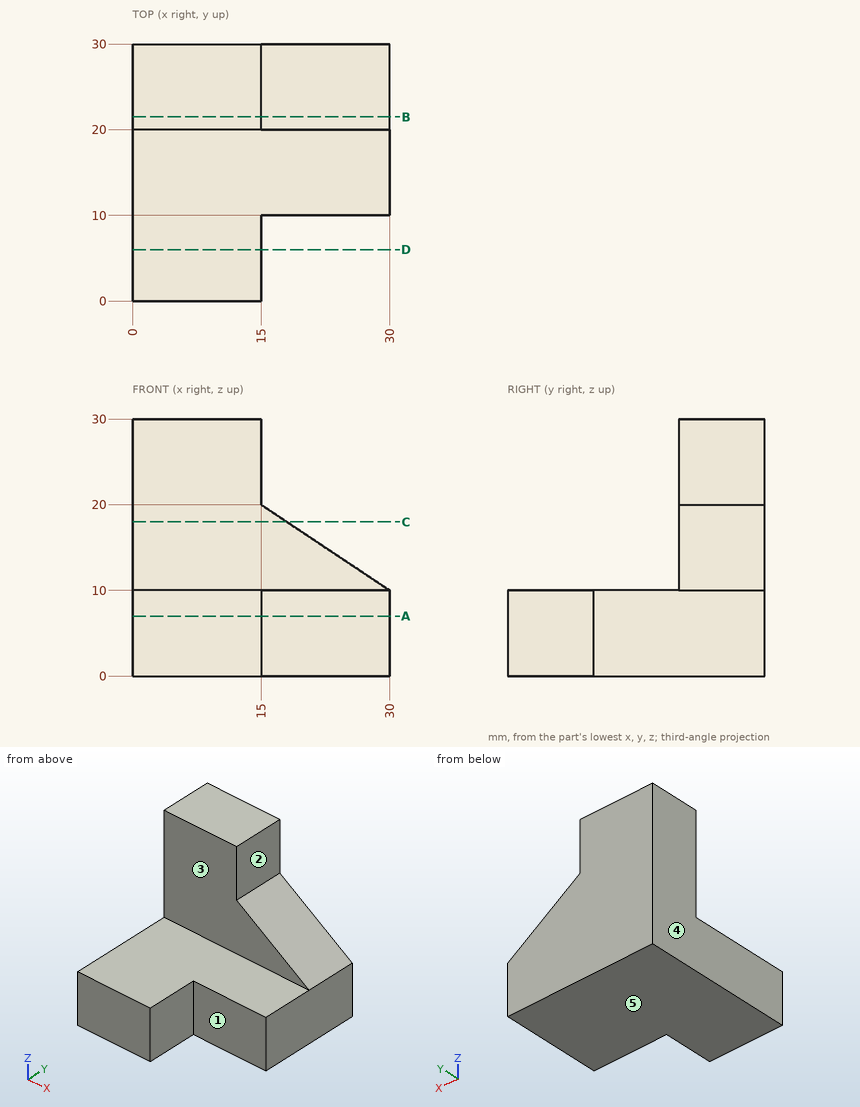
Design review of the part shown in the three views and the two pictorial views. Dimensions are in mm from the part's minimum x, y and z. A direction names the side the tool comes from. Give positions to 0.01 mm unless a question says otherwise; leave off trailing zeros. Loops run counter-clockwise (first coordinate to the right, second up) from the corner with the lowest first, then second, coordinate; pieces in that order, holes last. Notation, with made-up numbers: (4.5, 63.25) -> (21.5, 63.25) arc R9 ccw to (21.5, 79.25) -> close; hole circle Ø7 at (34.5, 63.5). An arc over 180 degrees is marked (long way). Put each result on its own line as item: value. Start each with the question number.
1. Clearance check with flat-ended pins moving along their axes: P1, Ø8, axis at y = 3, z = 6, coming from the +X side; P2, Ø11, axis at x = 21.5, z = 5, coming from the -Y side; P3, Ø1.5, axis at x = 18.5, y = 14.5, coming from the +Z side. State where each tip first meets the part, or that it passes through.
2. We need section B-B on y = 21.5. State the section outline as (x, z) points.
3. We need section A-A on z = 7. State the section outline as (x, y) points.
4. Wall thickness on probe 1 along Y at (x, z) = (26, 5); probe 2 along X at (y, z) = (28, 24.25); probe 3 along Y at (x, z) = (9.75, 25): over which ranges is each line inside the solid? List them lowest first.
5. We need section C-C on z = 18. State the section outline as (x, y) points, then the cut area to 3 significant figures.
6. For the marked faces 1, 2, 3, 4 and 5, list the 3-axis set-ups (+Z, -Z, +X, -X, +Y, -Y) from which the entire face can be reached by the end or side of a thin tool; tool diameter is ignored.
7. We need section D-D on y = 6. State the section outline as (x, z) points, then the cut area to 3 significant figures.
Determined:
1. P1: x = 15
1. P2: y = 10
1. P3: z = 10
2. outline: (0, 0) -> (30, 0) -> (30, 10) -> (15, 20) -> (15, 30) -> (0, 30) -> close
3. outline: (0, 0) -> (15, 0) -> (15, 10) -> (30, 10) -> (30, 30) -> (0, 30) -> close
4. probe 1: 10 to 30
4. probe 2: 0 to 15
4. probe 3: 20 to 30
5. outline: (0, 20) -> (18, 20) -> (18, 30) -> (0, 30) -> close
5. area: 180 mm^2
6. face 1: +Z, -Z, +X, -Y
6. face 2: +Z, +X, +Y, -Y
6. face 3: +Z, +X, -X, -Y
6. face 4: +Z, -Z, -X, +Y, -Y
6. face 5: -Z, +X, -X, +Y, -Y
7. outline: (0, 0) -> (15, 0) -> (15, 10) -> (0, 10) -> close
7. area: 150 mm^2
